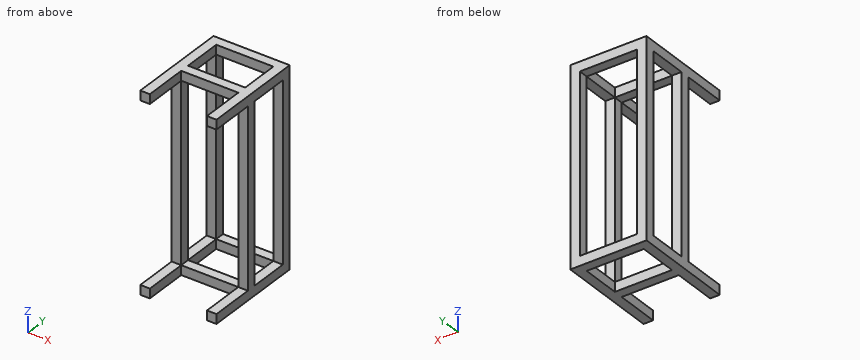
```python
from build123d import *

# Parameters (mm, degrees)
SKETCH1_W           = 480
SKETCH1_H           = 330
BOSS_EXTRUDE1_DEPTH = 80
SKETCH2_W           = 80
SKETCH2_H           = 80
BOSS_EXTRUDE2_DEPTH = 745


with BuildPart() as part:
    # Sketch1 → Boss-Extrude1 (new body)
    with BuildSketch(Plane.XY):
        Polygon((640, 0), (0, 0), (0, -857.8016), (80, -857.8016), (80, -490), (560, -490), (560, -857.8016), (640, -857.8016), align=None)
        with Locations((320, -245)):
            Rectangle(SKETCH1_W, SKETCH1_H, mode=Mode.SUBTRACT)
    boss_extrude1 = extrude(amount=-BOSS_EXTRUDE1_DEPTH)

    # Sketch2 → Boss-Extrude2 (add)
    with BuildSketch(Plane(origin=(0, 0, -80), x_dir=(-1, 0, 0), z_dir=(0, 0, -1))):
        with Locations((-600, -40)):
            Rectangle(SKETCH2_W, SKETCH2_H)
        with Locations((-40, -40)):
            Rectangle(SKETCH2_W, SKETCH2_H)
        with Locations((-600, -450)):
            Rectangle(SKETCH2_W, SKETCH2_H)
        with Locations((-40, -450)):
            Rectangle(SKETCH2_W, SKETCH2_H)
    boss_extrude2 = extrude(amount=BOSS_EXTRUDE2_DEPTH)

    # Mirror2: Boss-Extrude2 across plane
    add(boss_extrude2.mirror(Plane.XY.offset(-825)))

    # Mirror3: Boss-Extrude1 across plane
    add(boss_extrude1.mirror(Plane.XY.offset(-825)))


solid = part.part
```
Build history of the part. All positions in model axes, mm. Give positions to 0.01 mm unless a question says otherwise; leave off trailing zeros. Loops run counter-clockwise (first coordinate to the right, second up) from the corner with the lowest first, then second, coordinate; pieces in that order, holes last. Notation, with made-up numbers: (71, 5.5) - (93, 5.5) arc R7 cw to (93, 11.5) - close; hole circle Ø3 at (9.5, 30.5). An arc over 180 degrees is marked (long way). Use a Markdown table: item, result.
(1) Drop a flat-ended pin along its axis: pin 1 Ø24 at (x, z) = (299.5, -1594) entering from -Y. Give the stop position or say it passes through.
Taken from the geometry:
| item | result |
|---|---|
| pin 1 | y = -490 |
(2) Wall check: line 1 along Y through (x, z) = (410.5, -73.5); line 2 along Z through (x, y) = (305, -422). Give the ranges that are in metal, low to high.
Taken from the geometry:
| item | result |
|---|---|
| line 1 | -490 to -410, -80 to 0 |
| line 2 | -1650 to -1570, -80 to 0 |
(3) Band-saw the part on C-C (x = 586). Give the cut face in (y, z), and give its area (3 significant figures).
Taken from the geometry:
| item | result |
|---|---|
| outline | (-857.8, -1650) - (0, -1650) - (0, 0) - (-857.8, 0) - (-857.8, -80) - (-490, -80) - (-490, -1570) - (-857.8, -1570) - close; hole (-410, -1570) - (-80, -1570) - (-80, -80) - (-410, -80) - close |
| area | 376,000 mm2 |
(4) Band-saw the part on B-B (y = -735). Give the cut face in (x, z), and give its area (3 significant figures).
Taken from the geometry:
| item | result |
|---|---|
| outline | (0, -1650) - (80, -1650) - (80, -1570) - (0, -1570) - close; (0, -80) - (80, -80) - (80, 0) - (0, 0) - close; (560, -1650) - (640, -1650) - (640, -1570) - (560, -1570) - close; (560, -80) - (640, -80) - (640, 0) - (560, 0) - close |
| area | 25,600 mm2 |
(5) Band-saw the part on A-A (x = 203.5). Give the cut face in (y, z).
Taken from the geometry:
| item | result |
|---|---|
| outline | (-490, -1650) - (-410, -1650) - (-410, -1570) - (-490, -1570) - close; (-490, -80) - (-410, -80) - (-410, 0) - (-490, 0) - close; (-80, -1650) - (0, -1650) - (0, -1570) - (-80, -1570) - close; (-80, -80) - (0, -80) - (0, 0) - (-80, 0) - close |
